```python
from build123d import *

# Parameters (mm, degrees)
MODEL_W             = 272
MODEL_H             = 84
MODEL_R             = 1.5
MODEL_W_2           = 12.5
MODEL_W_3           = 17
MODEL_H_2           = 28
BOSS_EXTRUDE1_DEPTH = 2


with BuildPart() as part:
    # Model → Boss-Extrude1 (new body)
    # profile 1 of 3: a face of its own
    with BuildSketch(Plane.XY):
        Rectangle(MODEL_W, MODEL_H)
        with Locations((-132, 26.75)):
            Circle(MODEL_R, mode=Mode.SUBTRACT)
        with Locations((-132, -36.25)):
            Circle(MODEL_R, mode=Mode.SUBTRACT)
        with Locations((132, -36.25)):
            Circle(MODEL_R, mode=Mode.SUBTRACT)
        with Locations((132, 10.75)):
            Circle(MODEL_R, mode=Mode.SUBTRACT)
        with Locations((132, 26.75)):
            Circle(MODEL_R, mode=Mode.SUBTRACT)
        with Locations((132, 36.25)):
            Circle(MODEL_R, mode=Mode.SUBTRACT)
        with Locations((-132, 10.75)):
            Circle(MODEL_R, mode=Mode.SUBTRACT)
        with Locations((-132, 36.25)):
            Circle(MODEL_R, mode=Mode.SUBTRACT)
    # profile 2 of 3: a face of its own
    with BuildSketch(Plane.XY):
        with Locations((-142.25, 0)):
            Rectangle(MODEL_W_2, MODEL_H)
    # profile 3 of 3: a face of its own
    with BuildSketch(Plane.XY):
        with Locations((-157, 0)):
            Rectangle(MODEL_W_3, MODEL_H_2)
    extrude(amount=BOSS_EXTRUDE1_DEPTH)


solid = part.part
```
Work out the finished part from the listing and answer in its coordinate system (mm). Coordinates: 2 decimals unless noted, no trailing zeros. Answer as a JSON object with one key per item and string values.
Q1. Given pin 1 Ø1.8 at (x, y) = (132, -36.25) entering from -Z; pin 2 Ø1 at (y, z) = (30.5, 0.5) entering from -X, each flat-ended and moving along its own axis, determine where each tip first touches the part or whether it passes through.
Results list:
{"pin 1": "passes through", "pin 2": "stops at x = -148.5"}
Q2. Find section A-A (z = 0.75). State how many separate pieces and enclosed holes the cut face has, plus the area to 3 significant figures.
Results list:
{"separate pieces": "1", "enclosed holes": "8", "area": "24,300 mm^2"}
Q3. Consider L1, parallel to Y at x = 132, z = 0.8; L2, parallel to X at y = 10.5, z = 0.4; L3, parallel to X at y = 9.5, z = 1.05. Determine where each line is inside the solid, lowest interval first. Write a range as from..to.
Results list:
{"L1": "y = -42..-37.75, -34.75..9.25, 12.25..25.25, 28.25..34.75, 37.75..42", "L2": "x = -165.5..-133.48, -130.52..130.52, 133.48..136", "L3": "x = -165.5..-132.83, -131.17..131.17, 132.83..136"}
